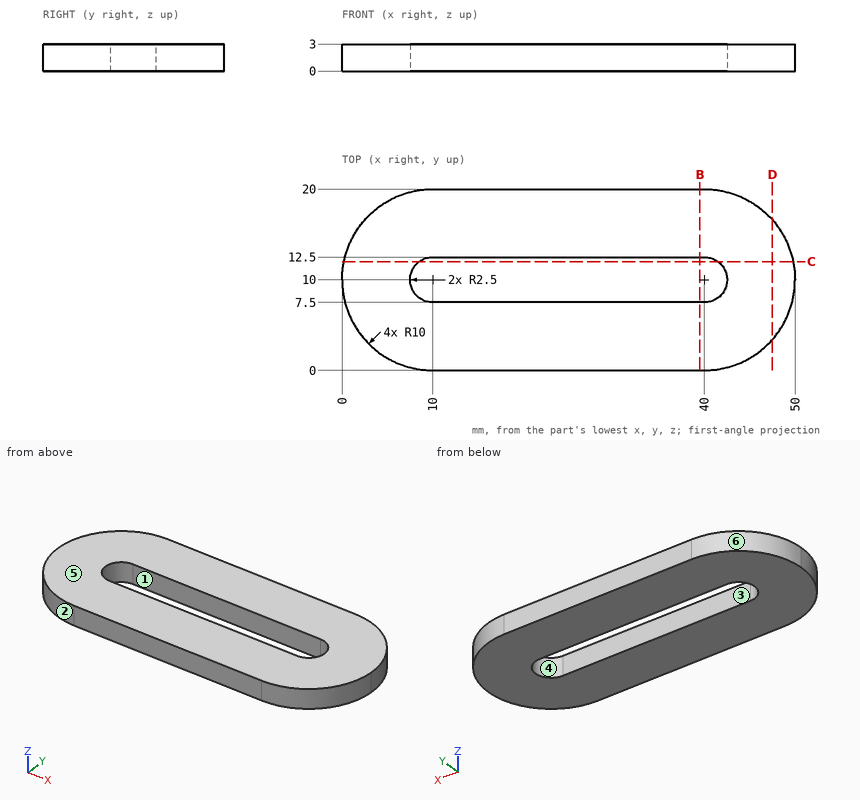
Geometry check sheet. Reference: drawing and pictorial views, mm from the part's lowest x, y, z. A direction names the side the tool comes from. Coordinates: 2 decimals unless noted, no trailing zeros. Write each loop counter-clockwise with the first axis right and the second up, starting at its lowest first coordinate (ties: lowest second). Pieces come first, ordered by that corner, then holes. Notation, with made-up numbers: (7, 11.5) -> (15, 11.5) arc R21 ccw to (15, 36.5) -> close; hole circle Ø1 at (-24, -24.5). An arc over 180 degrees is marked (long way). One line per question, with ' | ' between items.
1. Draft check along Y on the marked faces 3, 4, 5 and 6. Enter one of: +Y half, -Y half, draft (parallel to the pull), parting line (faces both ways), or undercut.
Answers:
face 3: undercut | face 4: undercut | face 5: draft | face 6: +Y half
2. Depth check by flat-ended pin: pin 1 Ø0.9 at (x, z) = (31.5, 1.5) entering from -Y; pin 2 Ø3 at (x, y) = (33.5, 10.5) entering from -Z. Enter the tip coordinate at first touch or a pass-through.
Answers:
pin 1: stops at y = 0 | pin 2: passes through
3. Cross-section at C-C on y = 12. Record the cut outline in (x, z).
Answers:
outline: (0.2, 0) -> (8.5, 0) -> (8.5, 3) -> (0.2, 3) -> close; (41.5, 0) -> (49.8, 0) -> (49.8, 3) -> (41.5, 3) -> close
4. Thickness scan on probe 1 along Y at (x, z) = (10, 1.85); probe 2 along X at (y, z) = (10.5, 2.25); probe 3 along X at (y, z) = (8.5, 1.25). Record the ranges inside material, lowest first. Write a range as from..to.
Answers:
probe 1: y = 0..7.5, 12.5..20 | probe 2: x = 0.01..7.55, 42.45..49.99 | probe 3: x = 0.11..8, 42..49.89
5. Cross-section at B-B on x = 39.5. Record the cut outline in (y, z), and give its area (3 significant figures).
Answers:
outline: (0, 0) -> (7.5, 0) -> (7.5, 3) -> (0, 3) -> close; (12.5, 0) -> (20, 0) -> (20, 3) -> (12.5, 3) -> close | area: 45.0 mm²
6. Set-up check for the marked faces 1 and 2: record each of +Z, -Z, +X, -X, +Y, -Y from which the full face is reachable in a straight line by a thin tool's end or side.
Answers:
face 1: +Z, -Z | face 2: +Z, -Z, -X, -Y
7. Cross-section at D-D on x = 47.5. Record the cut outline in (y, z), and give its area (3 significant figures).
Answers:
outline: (3.39, 0) -> (16.61, 0) -> (16.61, 3) -> (3.39, 3) -> close | area: 39.7 mm²
